from build123d import *

# Parameters (mm, degrees)
SKETCH_1_R          = 14
EXTRUDE_1_DEPTH     = 3
SKETCH_2_R          = 12.4
EXTRUDE_2_DEPTH     = 7
SKETCH_3_R          = 1.65
CUT_EXTRUDE_1_DEPTH = 5.1
SKETCH_4_R          = 3.5
CUT_EXTRUDE_2_DEPTH = 11
SKETCH_6_R          = 1.95
CUT_EXTRUDE_4_DEPTH = 3.2
CHAMFER_1_SIZE      = 0.5


with BuildPart() as part:
    # 草图1 → 凸台-拉伸1 (new body)
    with BuildSketch(Plane(origin=(0, 0, 0), x_dir=(1, 0, 0), z_dir=(0, 1, 0))):
        Circle(SKETCH_1_R)
    extrude(amount=EXTRUDE_1_DEPTH)

    # 草图2 → 凸台-拉伸2 (add)
    with BuildSketch(Plane(origin=(0, 3, 0), x_dir=(1, 0, 0), z_dir=(0, 1, 0))):
        Circle(SKETCH_2_R)
    extrude(amount=EXTRUDE_2_DEPTH)

    # 草图3 → 切除-拉伸1 (cut)
    with BuildSketch(Plane.XZ):
        with Locations((10.5, 0)):
            Circle(SKETCH_3_R)
        with Locations((5.25, -9.09326674)):
            Circle(SKETCH_3_R)
        with Locations((-5.25, -9.09326674)):
            Circle(SKETCH_3_R)
        with Locations((-10.5, 0)):
            Circle(SKETCH_3_R)
        with Locations((-5.25, 9.09326674)):
            Circle(SKETCH_3_R)
        with Locations((5.25, 9.09326674)):
            Circle(SKETCH_3_R)
    extrude(amount=-CUT_EXTRUDE_1_DEPTH, mode=Mode.SUBTRACT)

    # 草图4 → 切除-拉伸2 (cut, through all)
    with BuildSketch(Plane.XZ):
        Circle(SKETCH_4_R)
    extrude(amount=-CUT_EXTRUDE_2_DEPTH, mode=Mode.SUBTRACT)

    # 草图6 → 切除-拉伸4 (cut)
    with BuildSketch(Plane(origin=(0, 10, 0), x_dir=(1, 0, 0), z_dir=(0, 1, 0))):
        with Locations((9, 0)):
            Circle(SKETCH_6_R)
        with Locations((-4.5, -7.794228634)):
            Circle(SKETCH_6_R)
        with Locations((-4.5, 7.794228634)):
            Circle(SKETCH_6_R)
    extrude(amount=-CUT_EXTRUDE_4_DEPTH, mode=Mode.SUBTRACT)

    # 倒角1
    chamfer_1_edges = [part.edges().sort_by_distance(p)[0] for p in [
        (7.05, 10, 0),
        (-6.45, 10, 7.794228634),
        (-6.45, 10, -7.794228634),
        (-12.4, 10, 0),
    ]]
    chamfer(chamfer_1_edges, length=CHAMFER_1_SIZE)


solid = part.part
Here's how the part is built. I have some questions about the finished solid (model axes, mm). A direction names the side the tool comes from. Give positions to 0.01 mm unless a question says otherwise; leave off trailing zeros. Order: outer loops, then holes, each group sorted by start corner. A loop starts at its lowest first (then second) coordinate and runs counter-clockwise, first axis right, second up. Notation, with made-up numbers: (-27.5, 57.25) -> (-14.5, 57.25) arc R14 cw to (-14.5, 72.25) -> close; hole circle Ø3 at (-34.5, 24.25). An arc over 180 degrees is marked (long way). One line per item, written item: value. Start each with the question number.
1. Imagine slicing it at B-B, the plane x = 0. List the corners of the cut face in (y, z) for me.
2. For faces 1 (the face through (5, 5.1, -9)), 2 (the face through (-5.94, 8.17, 6.48)), which set-ups out of +Z, -Z, +X, -X, +Y, -Y let a thin tool reach every point of the face, with its end or its side?
3. Will these pins go through, and if not, where does the flat tip stop? pin 1 Ø1.2 at (x, z) = (-4, 8) entering from +Y; pin 2 Ø1.5 at (y, z) = (4.5, 4) entering from +X; pin 3 Ø4 at (y, z) = (6.5, 9.5) entering from -X.
4. I need wall thicknesses on probe 1 along Z at (x, y) = (6, 3.5); probe 2 along Z at (x, y) = (-4.5, 7.55); probe 3 along Z at (x, y) = (0, 4). Which ranges of each line are inside material? Lowest first, please. Write a range as from..to.
5. Imagine slicing it at C-C, the plane y = 5.5. List the corners of the cut face in (x, z) for me.
6. We'd pull the mould along X, two halves only. Please class faces 3 (the face through (-6.47, 2.51, -7.98)), 4 (the face through (3, 0, 3)), 5 (the face through (5.72, 6.2, 11)): released by +X, released by -X, zero draft, split by the parting line, or undercut.
7. Imagine slicing it at A-A, the plane z = 0. List the corners of the cut face in (x, y) for me.
Values follow:
1. outline: (0, -14) -> (3, -14) -> (3, -12.4) -> (9.5, -12.4) -> (10, -11.9) -> (10, -3.5) -> (0, -3.5) -> close; (0, 3.5) -> (10, 3.5) -> (10, 11.9) -> (9.5, 12.4) -> (3, 12.4) -> (3, 14) -> (0, 14) -> close
2. face 1: -Y
2. face 2: +Y
3. pin 1: stops at y = 6.8
3. pin 2: stops at x = 11.97
3. pin 3: stops at x = -9.87
4. probe 1: z = -10.85..-10.56, -7.62..7.62, 10.56..10.85
4. probe 2: z = -11.55..-9.74, -5.84..5.84, 9.74..11.55
4. probe 3: z = -12.4..-3.5, 3.5..12.4
5. outline: circle Ø24.8 at (0, 0); hole circle Ø7 at (0, 0)
6. face 3: undercut
6. face 4: zero draft
6. face 5: split by the parting line
7. outline: (-14, 0) -> (-12.15, 0) -> (-12.15, 5.1) -> (-8.85, 5.1) -> (-8.85, 0) -> (-3.5, 0) -> (-3.5, 10) -> (-11.9, 10) -> (-12.4, 9.5) -> (-12.4, 3) -> (-14, 3) -> close; (3.5, 0) -> (8.85, 0) -> (8.85, 5.1) -> (12.15, 5.1) -> (12.15, 0) -> (14, 0) -> (14, 3) -> (12.4, 3) -> (12.4, 9.5) -> (11.9, 10) -> (11.45, 10) -> (10.95, 9.5) -> (10.95, 6.8) -> (7.05, 6.8) -> (7.05, 9.5) -> (6.55, 10) -> (3.5, 10) -> close
